Here's how the part is built. I have some questions about the finished solid (model axes, mm). A direction names the side the tool comes from. Round coordinates to 2 decimals unless told otherwise and drop trailing zeros. Loops run counter-clockwise (first coordinate to the right, second up) from the corner with the lowest first, then second, coordinate; pieces in that order, holes last. Notation, with made-up numbers: (9, 32) -> (44, 32) arc R32 ccw to (44, 60) -> close; hole circle Ø1 at (49.25, 24). An arc over 180 degrees is marked (long way). Use CSV: the item, a comma, the result in double quotes. Start each with the question number.
from build123d import *

# Parameters (mm, degrees)
SKETCH1_R           = 18.5
BOSS_EXTRUDE1_DEPTH = 70
SKETCH2_R           = 5.969
BOSS_EXTRUDE2_DEPTH = 6.096
SKETCH3_R           = 3.048
BOSS_EXTRUDE3_DEPTH = 16.002
SKETCH4_R           = 1.6
CUT_EXTRUDE1_DEPTH  = 3


with BuildPart() as part:
    # Sketch1 → Boss-Extrude1 (new body)
    with BuildSketch(Plane.XY):
        Circle(SKETCH1_R)
    extrude(amount=BOSS_EXTRUDE1_DEPTH)

    # Sketch2 → Boss-Extrude2 (add)
    with BuildSketch(Plane(origin=(0, 0, 0), x_dir=(-1, 0, 0), z_dir=(0, 0, -1))):
        with Locations((0, -7.112)):
            Circle(SKETCH2_R)
    extrude(amount=BOSS_EXTRUDE2_DEPTH)

    # Sketch3 → Boss-Extrude3 (add)
    with BuildSketch(Plane(origin=(0, 0, -6.096), x_dir=(-1, 0, 0), z_dir=(0, 0, -1))):
        with Locations((0, -7.112)):
            Circle(SKETCH3_R)
    extrude(amount=BOSS_EXTRUDE3_DEPTH)

    # Sketch4 → Cut-Extrude1 (cut)
    with BuildSketch(Plane(origin=(0, 0, 0), x_dir=(-1, 0, 0), z_dir=(0, 0, -1))):
        with Locations((-15.2766, 0)):
            Circle(SKETCH4_R)
        with Locations((15.2766, 0)):
            Circle(SKETCH4_R)
        with Locations((7.794229315, -13.567540858)):
            Circle(SKETCH4_R)
        with Locations((-7.794229315, -13.567540858)):
            Circle(SKETCH4_R)
        with Locations((-7.794229315, 13.214096537)):
            Circle(SKETCH4_R)
        with Locations((7.794229315, 13.214096537)):
            Circle(SKETCH4_R)
    extrude(amount=-CUT_EXTRUDE1_DEPTH, mode=Mode.SUBTRACT)


solid = part.part
Q1. I need wall thicknesses on line 1 along Y through (x, z) = (-0.5, 56.5); line 2 along Z through (x, y) = (0, -12.5); line 3 along Z through (x, y) = (5, 6). Which ranges of each line are inside material? Lowest first, please.
Q2. I want a section at B-B, the plane y = 0. List the corners of the cut face in (x, z) for me, then the cut area to 3 significant figures.
Q3. For faces 1 (the flat face through (0, -7, -22.098)), 2 (the cylindrical face through (0.777, -1.194, -3.005)), which set-ups out of +Z, -Z, +X, -X, +Y, -Y let a thin tool reach every point of the face, with its end or its side?
Q4. If we mould it in two halves opening along X, with no side actions, what happens to faces 3 (the flat face through (3, -6, -6.096)), 4 (the cylindrical face through (7.056, 11.795, 1.479)), 5 (the cylindrical face through (0.4, -4.09, -13.98))? For each: pulls with the +X half, pulls with the -X half, needs draft (parallel to the pull), parting line crosses it, or undercut.
Q5. Will these pins go through, and if not, where does the flat tip stop? pin 1 Ø2.5 at (x, y) = (-7, 13) entering from -Z; pin 2 Ø1.9 at (x, y) = (7.79, -13.57) entering from -Z; pin 3 Ø11 at (x, y) = (1.5, 2.5) entering from -Z.
Q6. I want a section at A-A, the plane x = 0. List the corners of the cut face in (y, z) for me.
Q7. I want a section at C-C, the plane z = 25. List the corners of the cut face in (x, y) for me, then the cut area to 3 significant figures.
Values found:
1,line 1,"-18.49 to 18.49"
1,line 2,"-6.1 to 70"
1,line 3,"0 to 70"
2,outline,"(-18.5, 0) -> (-16.88, 0) -> (-16.88, 3) -> (-13.68, 3) -> (-13.68, 0) -> (13.68, 0) -> (13.68, 3) -> (16.88, 3) -> (16.88, 0) -> (18.5, 0) -> (18.5, 70) -> (-18.5, 70) -> close"
2,area,"2,570 mm2"
3,face 1,"-Z, +X, -X, +Y, -Y"
3,face 2,"-Z"
4,face 3,"needs draft"
4,face 4,"undercut"
4,face 5,"parting line crosses it"
5,pin 1,"z = 0"
5,pin 2,"z = 3"
5,pin 3,"z = -6.1"
6,outline,"(-18.5, 0) -> (-13.08, 0) -> (-13.08, -6.1) -> (-10.16, -6.1) -> (-10.16, -22.1) -> (-4.06, -22.1) -> (-4.06, -6.1) -> (-1.14, -6.1) -> (-1.14, 0) -> (18.5, 0) -> (18.5, 70) -> (-18.5, 70) -> close"
7,outline,"circle Ø37 at (0, 0)"
7,area,"1,080 mm2"
